Could you check a few things on this model? Use its own coordinates, in mm. A direction names the side the tool comes from. Give positions to 0.01 mm unless a question says otherwise; leave off trailing zeros. Loops run counter-clockwise (first coordinate to the right, second up) from the corner with the lowest first, then second, coordinate; pieces in that order, holes last.
1. I need wall thicknesses on line 1 along Y through (x, z) = (0, 7.5); line 2 along X through (y, z) = (0, 8.5); line 3 along X through (y, z) = (-4.5, 2.5). Which ranges of each line are inside material? Lowest first, please.
2. For faces 1 (the flat face through (25.5, -0.1, 2.982)), 2 (the cylindrical face through (-20.867, -16, 6.07)), 3 (the flat face through (-18, -18, 0)), which set-ups out of +Z, -Z, +X, -X, +Y, -Y let a thin tool reach every point of the face, with its end or its side?
3. Imagine slicing it at A-A (x = 0). List the corners of the cut face in (y, z) for me.
4. Imagine slicing it at B-B (y = 0). List the corners of the cut face in (x, z) for me, plus the area to 3 significant figures.
5. Imagine slicing it at C-C (z = 7.25). List the corners of the cut face in (x, y) for me, plus the area to 3 significant figures.
6. For P1, Ø1.1, axis at x = 25, y = 3.5, coming from the +Z side; P2, Ø1, axis at x = 20, z = 7.5, coming from the +Y side; P3, Ø3, axis at y = 18.5, z = 6, coming from the -X side, each with a flat end and sliding along its axis, tell me the tip position at first contact or that it passes through.
```python
from build123d import *

# Parameters (mm, degrees)
F0_W          = 1
F0_H          = 8.0183284022
F2_ANGLE_BACK = 18
F2_ANGLE      = 36


with BuildPart() as f1:
    # F0 (on Front) → F1 (revolve)
    with BuildSketch(Plane.XZ):
        Polygon((25.295096, 2.9816715978), (25.295096, 0), (27.295096, 0), (27.295096, 1), (26.295096, 1), (26.295096, 2.9816715978), align=None)
        with Locations((25.795096, 6.9908357989)):
            Rectangle(F0_W, F0_H)
    revolve(axis=Axis((0, 0, 8.8810138404), (0, 0, 1)))

    # F0 (on Front) → F2 (revolve, cut)
    with BuildSketch(Plane.XZ, mode=Mode.PRIVATE) as f2_sk:
        Polygon((17.5041668117, 2.9816715978), (25.295096, 2.9816715978), (25.295096, 11), (26.295096, 11), (26.295096, 2.9816715978), (28.2746478915, 2.9816715978), (28.2746478915, 12.9816715978), (17.5041668117, 12.9816715978), align=None)
        with Locations((25.795096, 6.9908357989)):
            Rectangle(F0_W, F0_H)
    revolve(f2_sk.sketch.rotate(Axis((0, 0, 8.8810138404), (0, 0, 1)), -F2_ANGLE_BACK), axis=Axis((0, 0, 8.8810138404), (0, 0, 1)), revolution_arc=F2_ANGLE, mode=Mode.SUBTRACT)


solid = f1.part
```
Derived:
1. line 1: y = -26.3 to -25.3, 25.3 to 26.3
1. line 2: x = -26.3 to -25.3
1. line 3: x = -25.91 to -24.89, 24.89 to 25.91
2. face 1: +Z, +X
2. face 2: +Z
2. face 3: -Z, +X, -X, +Y, -Y
3. outline: (-27.3, 0) - (-25.3, 0) - (-25.3, 11) - (-26.3, 11) - (-26.3, 1) - (-27.3, 1) - close; (25.3, 0) - (27.3, 0) - (27.3, 1) - (26.3, 1) - (26.3, 11) - (25.3, 11) - close
4. outline: (-27.3, 0) - (-25.3, 0) - (-25.3, 11) - (-26.3, 11) - (-26.3, 1) - (-27.3, 1) - close; (25.3, 0) - (27.3, 0) - (27.3, 1) - (26.3, 1) - (26.3, 2.98) - (25.3, 2.98) - close
4. area: 16.0 mm2
5. outline: (24.06, -7.82) arc R25.3 cw (long way) to (24.06, 7.82) - (25.01, 8.13) arc R26.3 ccw (long way) to (25.01, -8.13) - close
5. area: 146 mm2
6. P1: stops at z = 2.98
6. P2: stops at y = 17.64
6. P3: stops at x = -20.06
